Input: part model. Units: mm. Frame: model coordinates. A direction names the side the tool comes from. Round coordinates to 2 decimals unless told otherwise and drop trailing zeros. Loops run counter-clockwise (first coordinate to the right, second up) from the corner with the lowest first, then second, coordinate; pieces in that order, holes last. Notation, with made-up numbers: (48, 46.25) -> (76, 46.25) arc R18 cw to (76, 59.25) -> close; hole circle Ø2 at (59.5, 2). An arc over 180 degrees is marked (long way). Answer as a JSON object with one key per item and string values. Group by question number.
Item 1: Section query A-A on x = -4. Return loops of the section in (y, z), and give its area (3 significant figures).
Item 2: Section query B-B on z = 20. Return loops of the section in (x, y), and give its area (3 significant figures).
Item 3: Section query C-C on y = -4. Return loops of the section in (x, z), and give its area (3 significant figures).
Item 4: Pin query (flat end, axial travel): pin 1 (2 mm diameter, centred on x = 15.5, z = 59.5, fed in from -Y); pin 2 (3 mm diameter, centred on x = 27, y = -11.5, fed in from -Z); pin 3 (12 mm diameter, centred on y = -42.5, z = -7, fed in from -X). Return the tip coordinate at first contact, or that it passes through.
Item 5: Set-up query: faces 1 (the flat face through (-2, -45, 26.15)), 2 (the flat face through (-2, -45, -37.35)), 3 (the flat face through (0, 0, -3)), 4 (the flat face through (-17.476, -45, -6)), 5 (the flat face through (14.274, -45, -6)). Return all of +Z, -Z, +X, -X, +Y, -Y with unobstructed straight access to the full face (end or side cutting, diameter ignored); none if empty.
Item 6: Section query D-D on y = -37.5. Return loops of the section in (x, z), and give its area (3 significant figures).
Item 7: Material intervals for line 1 (Y direction, x = -10, z = -47); line 2 (Z direction, x = -5, y = -59); line 3 (Z direction, x = 29.5, y = -7.5), sorted ascending. Write a range as [from, to].
from build123d import *

# Parameters (mm, degrees)
F1_DEPTH = 25.4
F2_W     = 31.75
F2_H     = 63.5
F3_DEPTH = 39.624


with BuildPart() as f1:
    # F0 (on Front) → F1 (new body)
    with BuildSketch(Plane.XZ):
        Polygon((-32.678649, 41.369968), (-32.216675, -56.016259), (34.556333, -55.800427), (34.245424, 40.38674), (0, 77.908613), align=None)
    extrude(amount=F1_DEPTH)

    # F2 (on face) → F3 (join)
    with BuildSketch(Plane.XZ.offset(25.4)):
        with Locations((-1.600679, -5.599995)):
            Rectangle(F2_W, F2_H)
    extrude(amount=F3_DEPTH)


solid = f1.part
Solved:
{
 "1": {"outline": "(-65.02, -37.35) -> (-25.4, -37.35) -> (-25.4, -55.93) -> (0, -55.93) -> (0, 73.44) -> (-25.4, 73.44) -> (-25.4, 26.15) -> (-65.02, 26.15) -> close", "area": "5,800 mm²"},
 "2": {"outline": "(-32.58, -25.4) -> (-17.48, -25.4) -> (-17.48, -65.02) -> (14.27, -65.02) -> (14.27, -25.4) -> (34.31, -25.4) -> (34.31, 0) -> (-32.58, 0) -> close", "area": "2,960 mm²"},
 "3": {"outline": "(-32.68, 41.37) -> (-32.22, -56.02) -> (34.56, -55.8) -> (34.25, 40.39) -> (0, 77.91) -> close", "area": "7,710 mm²"},
 "4": {"pin 1": "y = -25.4", "pin 2": "z = -55.83", "pin 3": "x = -17.48"},
 "5": {"face 1": "+Z, +X, -X, -Y", "face 2": "-Z, +X, -X, -Y", "face 3": "+Z, -Z, +X, -X, +Y", "face 4": "+Z, -Z, -X, -Y", "face 5": "+Z, -Z, +X, -Y"},
 "6": {"outline": "(-17.48, -37.35) -> (14.27, -37.35) -> (14.27, 26.15) -> (-17.48, 26.15) -> close", "area": "2,020 mm²"},
 "7": {"line 1": "[-25.4, 0]", "line 2": "[-37.35, 26.15]", "line 3": "[-55.82, 45.59]"}
}
